from build123d import *

# Parameters (mm, degrees)
BOSS_EXTRUDE1_DEPTH   = 3.175
F_4_CLEARANCE_HOLE1_D = 2.9464
BOSS_EXTRUDE2_DEPTH   = 3.175


with BuildPart() as part:
    # Sketch1 → Boss-Extrude1 (new body)
    with BuildSketch(Plane(origin=(0, 0, -14.15699402), x_dir=(-1, 0, 0), z_dir=(0, 0, -1))):
        with BuildLine():
            Line((-49.172312317, -34.502108483), (-53.141062317, -27.628031841))
            ThreePointArc((-53.141062317, -27.628031841), (-55.063803638, -24.012221257), (-56.72992661, -20.271224785))
            ThreePointArc((-56.72992661, -20.271224785), (-54.976138042, -16.13776671), (-50.842679967, -17.891555277))
            ThreePointArc((-50.842679967, -17.891555277), (-49.356678398, -21.228119699), (-47.641801003, -24.453031841))
            Line((-47.641801003, -24.453031841), (-43.673051003, -31.327108483))
            ThreePointArc((-43.673051003, -31.327108483), (-16.68272836, -52.037511462), (17.046778195, -47.596937682))
            Line((17.046778195, -47.596937682), (23.920854837, -43.628187682))
            Line((23.920854837, -43.628187682), (30.79493148, -39.659437682))
            ThreePointArc((30.79493148, -39.659437682), (51.505334458, -12.669115038), (47.064760678, 21.060391517))
            Line((47.064760678, 21.060391517), (43.096010678, 27.934468159))
            ThreePointArc((43.096010678, 27.934468159), (41.160593535, 31.032051618), (39.01404477, 33.987248938))
            ThreePointArc((39.01404477, 33.987248938), (39.561948355, 38.44382292), (44.018522337, 37.895919335))
            ThreePointArc((44.018522337, 37.895919335), (46.425258832, 34.58251628), (48.595271992, 31.109468159))
            Line((48.595271992, 31.109468159), (52.564021992, 24.235391517))
            ThreePointArc((52.564021992, 24.235391517), (57.638963455, -14.312615975), (33.96993148, -45.158698996))
            Line((33.96993148, -45.158698996), (27.095854837, -49.127448996))
            Line((27.095854837, -49.127448996), (20.221778195, -53.096198996))
            ThreePointArc((20.221778195, -53.096198996), (-18.326229296, -58.171140459), (-49.172312317, -34.502108483))
        make_face()
    extrude(amount=BOSS_EXTRUDE1_DEPTH)

    # #4 Clearance Hole1 (through all)
    with Locations(Plane(origin=(0, 0, -17.33199402), x_dir=(-1, 0, 0), z_dir=(0, 0, -1))):
        with Locations((-53.56643166, -20.541270527), (-47.21643166, -31.539793155), (42.670641335, 35.021229473), (49.020641335, 24.022706845)):
            Hole(F_4_CLEARANCE_HOLE1_D / 2)

    # Sketch6 → Boss-Extrude2 (add)
    with BuildSketch(Plane.XY.offset(-14.15699402)):
        Polygon((60.420653285, -72.901641316), (32.924346715, -88.776641316), (13.712730754, -55.501146376), (41.209037324, -39.626146376), align=None)
        with BuildLine():
            Line((46.862720596, -59.172213053), (48.856620596, -62.625749158))
            ThreePointArc((48.856620596, -62.625749158), (44.831, -77.649569754), (29.807179404, -73.623949158))
            Line((29.807179404, -73.623949158), (27.813279404, -70.170413053))
            ThreePointArc((27.813279404, -70.170413053), (31.8389, -55.146592457), (46.862720596, -59.172213053))
        make_face(mode=Mode.SUBTRACT)
        with BuildLine():
            Line((33.866506919, -84.566510659), (31.872606919, -81.112974554))
            ThreePointArc((31.872606919, -81.112974554), (32.402538499, -79.135242974), (34.380270079, -79.665174554))
            Line((34.380270079, -79.665174554), (36.374170079, -83.118710659))
            ThreePointArc((36.374170079, -83.118710659), (35.844238499, -85.096442239), (33.866506919, -84.566510659))
        make_face(mode=Mode.SUBTRACT)
        with BuildLine():
            Line((22.874070079, -59.735851552), (24.867970079, -63.189387657))
            ThreePointArc((24.867970079, -63.189387657), (24.338038499, -65.167119237), (22.360306919, -64.637187657))
            Line((22.360306919, -64.637187657), (20.366406919, -61.183651552))
            ThreePointArc((20.366406919, -61.183651552), (20.896338499, -59.205919972), (22.874070079, -59.735851552))
        make_face(mode=Mode.SUBTRACT)
        with BuildLine():
            Line((42.803393081, -48.229651552), (44.797293081, -51.683187657))
            ThreePointArc((44.797293081, -51.683187657), (44.267361501, -53.660919237), (42.289629921, -53.130987657))
            Line((42.289629921, -53.130987657), (40.295729921, -49.677451552))
            ThreePointArc((40.295729921, -49.677451552), (40.825661501, -47.699719972), (42.803393081, -48.229651552))
        make_face(mode=Mode.SUBTRACT)
        with BuildLine():
            Line((54.309593081, -68.158974554), (56.303493081, -71.612510659))
            ThreePointArc((56.303493081, -71.612510659), (55.773561501, -73.590242239), (53.795829921, -73.060310659))
            Line((53.795829921, -73.060310659), (51.801929921, -69.606774554))
            ThreePointArc((51.801929921, -69.606774554), (52.331861501, -67.629042974), (54.309593081, -68.158974554))
        make_face(mode=Mode.SUBTRACT)
    extrude(amount=-BOSS_EXTRUDE2_DEPTH)


solid = part.part
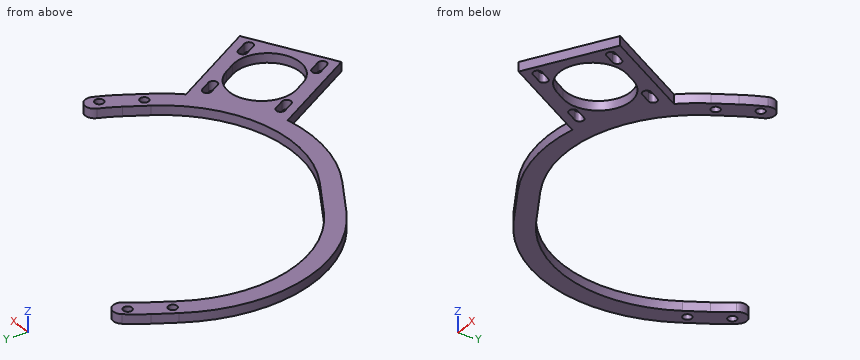
Design review of the part built by this model. Coordinates are the model's own, in mm. Give positions to 0.01 mm unless a question says otherwise; leave off trailing zeros. Write each loop counter-clockwise with the first axis right and the second up, starting at its lowest first coordinate (ties: lowest second). Pieces come first, ordered by that corner, then holes. Notation, with made-up numbers: M -38,-18.5 L -4,-18.5 A21 cw -4,2.5 Z; hole C 34,70 d10. An arc over 180 degrees is marked long. Answer as a JSON object with one key per item and string values. Group by question number.
1) We need section A-A (y = -36.5). Give the boundary of the cut face in (x, z).
2) For line 1 along Y through (x, z) = (-49.5, -14.4); line 2 along Y through (x, z) = (48.5, -16.65); line 3 along Y through (x, z) = (42.5, -17), list the stretches that pass through material, from the lowest coordinate up.
3) We need section C-C (x = -32.5). Give the boundary of the cut face in (y, z), and give its area (3 significant figures).
4) Clearance check with flat-ended pins moving along their axes: pin 1 Ø2.5 at (x, y) = (-42.67, 35.02) entering from -Z; pin 2 Ø1.5 at (y, z) = (-70, -14.5) entering from +X; pin 3 Ø1.5 at (x, z) = (-36, -15.5) entering from -Y; pin 4 Ø1 at (x, z) = (-16.5, -15.5) entering from +Y. State where each tip first meets the part, or that it passes through.
5) We need section D-D (y = 5.5). Give the boundary of the cut face in (x, z).
6) We need section B-B (z = -15). Count the separate pieces of the cut face and the enclosed holes in it, and give its area (3 significant figures).
Answer key:
{
 "1": {"outline": "M -45.07,-17.33 L -35.54,-17.33 L -35.54,-14.16 L -45.07,-14.16 Z; M 40.18,-17.33 L 47.96,-17.33 L 47.96,-14.16 L 40.18,-14.16 Z"},
 "2": {"line 1": "y = -31.25 to -18.5, 16.17 to 22.63, 25.42 to 29.54", "line 2": "y = -79.78 to -74.2, -62.01 to -52.25, -35.63 to -32.26, -30.82 to -22.91", "line 3": "y = -83.25 to -78.66, -54.96 to -53.41, -47.86 to -33.25"},
 "3": {"outline": "M -46.01,-17.33 L -38.62,-17.33 L -38.62,-14.16 L -46.01,-14.16 Z", "area": "23.4 mm²"},
 "4": {"pin 1": "passes through", "pin 2": "stops at x = 59.18", "pin 3": "stops at y = -44.39", "pin 4": "stops at y = -47.62"},
 "5": {"outline": "M -58.93,-17.33 L -52.52,-17.33 L -52.52,-14.16 L -58.93,-14.16 Z"},
 "6": {"separate pieces": "1", "enclosed holes": "9", "area": "1,760 mm²"}
}
